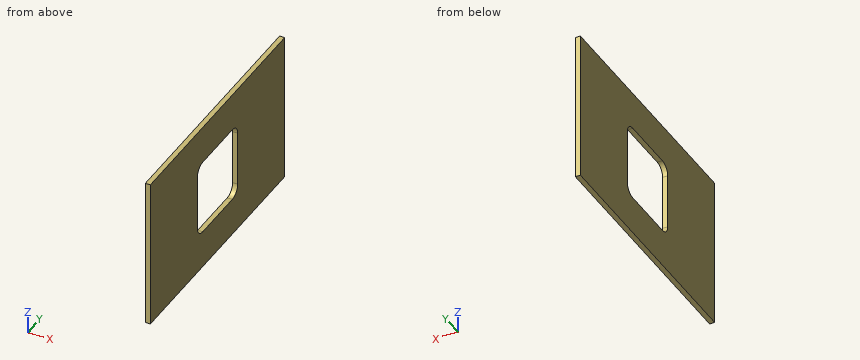
```python
from build123d import *

# Parameters (mm, degrees)
SKETCH1_W           = 500
SKETCH1_H           = 300
BOSS_EXTRUDE1_DEPTH = 10


with BuildPart() as part:
    # Sketch1 → Boss-Extrude1 (new body)
    with BuildSketch(Plane.YZ):
        with Locations((250, 150)):
            Rectangle(SKETCH1_W, SKETCH1_H)
        with BuildLine():
            Line((195, 75), (305, 75))
            ThreePointArc((305, 75), (319.142135624, 80.857864376), (325, 95))
            Line((325, 95), (325, 205))
            ThreePointArc((325, 205), (319.142135624, 219.142135624), (305, 225))
            Line((305, 225), (195, 225))
            ThreePointArc((195, 225), (180.857864376, 219.142135624), (175, 205))
            Line((175, 205), (175, 95))
            ThreePointArc((175, 95), (180.857864376, 80.857864376), (195, 75))
        make_face(mode=Mode.SUBTRACT)
    extrude(amount=BOSS_EXTRUDE1_DEPTH)


solid = part.part
```
Design review of the part built by this model. Coordinates are the model's own, in mm. Round coordinates to 2 decimals unless told otherwise and drop trailing zeros. Write each loop counter-clockwise with the first axis right and the second up, starting at its lowest first coordinate (ties: lowest second). Pieces come first, ordered by that corner, then holes.
Item 1: We need section B-B on y = 200. Write out the cut boundary in (x, z), and give its area (3 significant figures).
Item 2: We need section A-A on x = 3. Write out the cut boundary in (y, z).
Item 3: We need section C-C on z = 112.5. Write out the cut boundary in (x, y).
Item 4: For probe 1 along Y at (x, z) = (7, 104); probe 2 along Z at (x, y) = (6.5, 202); probe 3 along Z at (x, y) = (9, 308.5), list the stretches that pass through material, from the lowest coordinate up.
Returned:
1. outline: (0, 0) - (10, 0) - (10, 75) - (0, 75) - close; (0, 225) - (10, 225) - (10, 300) - (0, 300) - close
1. area: 1,500 mm2
2. outline: (0, 0) - (500, 0) - (500, 300) - (0, 300) - close; hole (175, 95) arc R20 ccw to (195, 75) - (305, 75) arc R20 ccw to (325, 95) - (325, 205) arc R20 ccw to (305, 225) - (195, 225) arc R20 ccw to (175, 205) - close
3. outline: (0, 0) - (10, 0) - (10, 175) - (0, 175) - close; (0, 325) - (10, 325) - (10, 500) - (0, 500) - close
4. probe 1: y = 0 to 175, 325 to 500
4. probe 2: z = 0 to 75, 225 to 300
4. probe 3: z = 0 to 75.31, 224.69 to 300
